Here's how the part is built. I have some questions about the finished solid (model axes, mm). Face numbers are marked on the shaded views. A direction names the side the tool comes from. Coordinates: 2 decimals unless noted, no trailing zeros. Write each loop counter-clockwise with the first axis right and the second up, starting at its lowest first coordinate (ties: lowest second). Pieces come first, ordered by that corner, then holes.
Item 1: I want a section at A-A (x = 3.25). Please give me the cut outline in (y, z).
Item 2: Please list where these lines run through material, in increasing order: line 1 (X direction, y = -5, z = 2.3); line 2 (Y direction, x = -4, z = 1.55); line 3 (Y direction, x = 12.5, z = 1.6).
Item 3: For the marked faces 4 and 5, which set-ups out of +Z, -Z, +X, -X, +Y, -Y let a thin tool reach every point of the face, with its end or its side?
Item 4: I want a section at D-D (y = 25). Please give me the cut outline in (x, z).
Item 5: I want a section at B-B (y = 14). Please give me the cut outline in (x, z).
Item 6: I'm going to push flat-ended pins straight in: P1, Ø2.5, axis at x = -10, y = 25, coming from the +Z side; P2, Ø6, axis at x = 9.5, y = 10, coming from the -Z side. Where does each tip first touch, or does it pass through?
Item 7: I want a section at C-C (z = 2.85). Please give me the cut outline in (x, y).
Item 8: If we mould it in two halves opening along X, with no side actions, what happens to the marked faces 1, 2 and 3? For each: pulls with the +X half, pulls with the -X half, needs draft (parallel to the pull), parting line crosses it, or undercut.
from build123d import *

# Parameters (mm, degrees)
SZKIC1_W                    = 28.8
SZKIC1_H                    = 60
DODANIE_WYCI_GNI_CIE1_DEPTH = 5
ZAOKR_GLENIE1_R             = 2
OTW_R_POD_RUB_M22_D         = 2.6
WYTNIJ_WYCI_GNI_CIE1_REACH  = 7


with BuildPart() as part:
    # Szkic1 → Dodanie-wyciągnięcie1 (new body)
    with BuildSketch(Plane.XY):
        Rectangle(SZKIC1_W, SZKIC1_H)
    extrude(amount=DODANIE_WYCI_GNI_CIE1_DEPTH)

    # Zaokrąglenie1
    zaokr_glenie1_edges = [part.edges().sort_by_distance(p)[0] for p in [
        (14.4, -30, 2.5),
        (-14.4, -30, 2.5),
        (-14.4, 30, 2.5),
        (14.4, 30, 2.5),
    ]]
    fillet(zaokr_glenie1_edges, radius=ZAOKR_GLENIE1_R)

    # Otwór pod śrubę M22 (through all)
    with Locations(Plane.XY.offset(5)):
        with Locations((10, 25), (10, -25), (-10, -25), (-10, 25)):
            Hole(OTW_R_POD_RUB_M22_D / 2)

    # Szkic7 → Wytnij-wyciągnięcie1 (cut, up to next)
    with BuildSketch(Plane.XY.offset(5), mode=Mode.PRIVATE) as wytnij_wyci_gni_cie1_sk1:
        with BuildLine():
            Line((5, 20), (-5, 20))
            ThreePointArc((-5, 20), (-8.535533906, 18.535533906), (-10, 15))
            Line((-10, 15), (-10, -15))
            ThreePointArc((-10, -15), (-8.535533906, -18.535533906), (-5, -20))
            Line((-5, -20), (5, -20))
            ThreePointArc((5, -20), (8.535533906, -18.535533906), (10, -15))
            Line((10, -15), (10, 15))
            ThreePointArc((10, 15), (8.535533906, 18.535533906), (5, 20))
        make_face()
    wytnij_wyci_gni_cie1_tool1 = extrude(wytnij_wyci_gni_cie1_sk1.sketch, amount=-WYTNIJ_WYCI_GNI_CIE1_REACH, mode=Mode.PRIVATE) & part.part
    add(wytnij_wyci_gni_cie1_tool1.solids().sort_by_distance((0, 0, 5))[0], mode=Mode.SUBTRACT)


solid = part.part
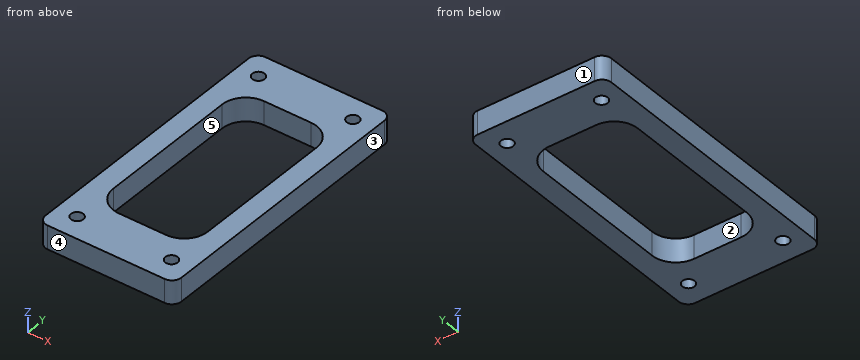
Answer:
1. outline: (-30, 0) - (-20, 0) - (-20, 5) - (-30, 5) - close; (20, 0) - (30, 0) - (30, 5) - (20, 5) - close
2. line 1: x = -14.4 to -10, 10 to 14.4
2. line 2: y = -30 to -20, 20 to 30
2. line 3: y = -30 to 30
3. face 4: +Z, -Z, +X, -X, -Y
3. face 5: +Z, -Z
4. outline: (-14.4, 0) - (-11.3, 0) - (-11.3, 5) - (-14.4, 5) - close; (-8.7, 0) - (8.7, 0) - (8.7, 5) - (-8.7, 5) - close; (11.3, 0) - (14.4, 0) - (14.4, 5) - (11.3, 5) - close
5. outline: (-14.4, 0) - (-10, 0) - (-10, 5) - (-14.4, 5) - close; (10, 0) - (14.4, 0) - (14.4, 5) - (10, 5) - close
6. P1: passes through
6. P2: stops at z = 0
7. outline: (-14.4, -28) arc R2 ccw to (-12.4, -30) - (12.4, -30) arc R2 ccw to (14.4, -28) - (14.4, 28) arc R2 ccw to (12.4, 30) - (-12.4, 30) arc R2 ccw to (-14.4, 28) - close; hole circle Ø2.6 at (-10, -25); hole circle Ø2.6 at (-10, 25); hole (-10, -15) arc R5 ccw to (-5, -20) - (5, -20) arc R5 ccw to (10, -15) - (10, 15) arc R5 ccw to (5, 20) - (-5, 20) arc R5 ccw to (-10, 15) - close; hole circle Ø2.6 at (10, -25); hole circle Ø2.6 at (10, 25)
8. face 1: needs draft
8. face 2: undercut
8. face 3: pulls with the +X half
